For this review, take the finished solid that the model builds, in its own axes (mm). Coordinates: 2 decimals unless noted, no trailing zeros. Loops run counter-clockwise (first coordinate to the right, second up) from the corner with the lowest first, then second, coordinate; pieces in that order, holes last.
1. Take a section at C-C, the plane x = 51. State the section outline as (y, z) points, then the cut area to 3 significant figures.
2. Take a section at B-B, the plane y = 9. State the section outline as (x, z) points.
3. Clearance check with flat-ended pins moving along their axes: P1, Ø1.5, axis at y = 11, z = 8.5, coming from the -X side; P2, Ø6, axis at y = -19, z = 9, coming from the -X side; P3, Ø2, axis at y = 14, z = 6, coming from the -X side. State where each tip first meets the part, or that it passes through.
4. Take a section at A-A, the plane z = 1.5. State the section outline as (x, y) points.
5. To check wall thickness, follow probe 1 along X at (y, z) = (-26, 5); probe 2 along X at (y, z) = (3.5, 1.75); probe 3 along Y at (x, z) = (-53.5, 4.5). State the ranges of each line that lie inside material, in increasing order.
```python
from build123d import *

# Parameters (mm, degrees)
F0_W     = 78.2
F0_H     = 60
F1_DEPTH = 10


with BuildPart() as f1:
    # F0 (on Top) → F1 (new body)
    with BuildSketch(Plane.XY):
        Polygon((59.099942, -29.952), (39.1, 30), (39.1, -30), align=None)
        Rectangle(F0_W, F0_H)
        with BuildLine():
            Line((-39.1, -30), (-39.1, 30))
            ThreePointArc((-39.1, 30), (-69.1, 0), (-39.1, -30))
        make_face()
    extrude(amount=F1_DEPTH)


solid = f1.part
```
Results list:
1. outline: (-29.97, 0) - (-5.67, 0) - (-5.67, 10) - (-29.97, 10) - close
1. area: 243 mm2
2. outline: (-67.72, 0) - (46.11, 0) - (46.11, 10) - (-67.72, 10) - close
3. P1: stops at x = -67.29
3. P2: stops at x = -64.48
3. P3: stops at x = -66.14
4. outline: (-39.1, -30) - (39.1, -30) - (59.1, -29.95) - (39.1, 30) - (-39.1, 30) arc R30 ccw to start
5. probe 1: x = -54.07 to 57.78
5. probe 2: x = -68.9 to 47.94
5. probe 3: y = -26.32 to 26.32
